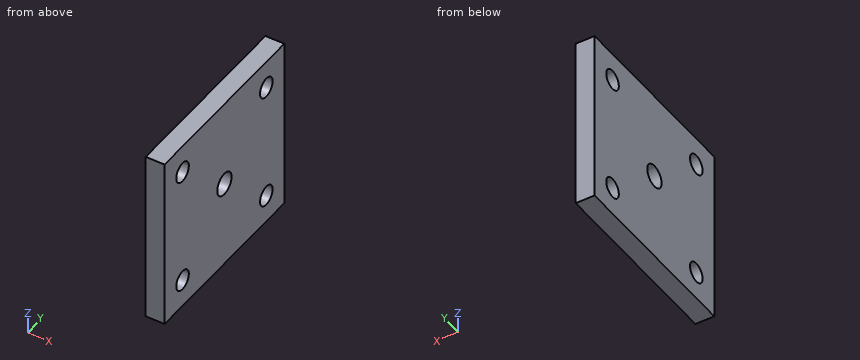
from build123d import *

# Parameters (mm, degrees)
F0_W     = 100
F0_H     = 93
F1_DEPTH = 10
F3_D     = 10.5
F4_D     = 12


with BuildPart() as f1:
    # F0 (on Right) → F1 (new body)
    with BuildSketch(Plane.YZ):
        with Locations((8.67743, 4.971333)):
            Rectangle(F0_W, F0_H)
    extrude(amount=F1_DEPTH)

    # F3 (through all)
    with Locations(Plane.YZ.offset(10)):
        with Locations((-26.32257, 36.471333), (43.67743, 36.471333), (-26.32257, -26.528667), (43.67743, -26.528667)):
            Hole(F3_D / 2)

    # F4 (through all)
    with Locations(Plane.YZ.offset(10)):
        with Locations((8.67743, 4.971333)):
            Hole(F4_D / 2)


solid = f1.part
Read the model definition and answer for the solid it produces. Units are mm, in the model's axes. Coordinates: 2 decimals unless noted, no trailing zeros. Order: outer loops, then holes, each group sorted by start corner. A loop starts at its lowest first (then second) coordinate and runs counter-clockwise, first axis right, second up. Notation, with made-up numbers: M -12,9 L 31,9 A13 cw 31,28 Z; hole C 87.25,70.5 d4. An arc over 180 degrees is marked long. Put each result on its own line as item: value. Start each with the question number.
Item 1: Section C-C, the plane x = 5.5 is taken. Determine the outline of the cut face in (y, z).
Item 2: Consider probe 1 along Y at (x, z) = (6, 37); probe 2 along Z at (x, y) = (7.25, 42); probe 3 along Y at (x, z) = (2.25, -28). Determine where each line is inside the solid, lowest interval first. Write a range as [from, to].
Item 3: Section A-A, the plane y = 40 is taken. Determine the outline of the cut face in (x, z).
Item 4: Section D-D, the plane y = 7.5 is taken. Determine the outline of the cut face in (x, z), plus the area to 3 significant figures.
Item 5: Section B-B, the plane z = 39.5 is taken. Determine the outline of the cut face in (x, y).
Computed:
1. outline: M -41.32,-41.53 L 58.68,-41.53 L 58.68,51.47 L -41.32,51.47 Z; hole C -26.32,-26.53 d10.5; hole C -26.32,36.47 d10.5; hole C 8.68,4.97 d12; hole C 43.68,-26.53 d10.5; hole C 43.68,36.47 d10.5
2. probe 1: y = [-41.32, -31.55], [-21.1, 38.45], [48.9, 58.68]
2. probe 2: z = [-41.53, -31.5], [-21.55, 31.5], [41.45, 51.47]
2. probe 3: y = [-41.32, -31.36], [-21.28, 38.64], [48.72, 58.68]
3. outline: M 0,-41.53 L 10,-41.53 L 10,-30.28 L 0,-30.28 Z; M 0,-22.78 L 10,-22.78 L 10,32.72 L 0,32.72 Z; M 0,40.22 L 10,40.22 L 10,51.47 L 0,51.47 Z
4. outline: M 0,-41.53 L 10,-41.53 L 10,-0.91 L 0,-0.91 Z; M 0,10.85 L 10,10.85 L 10,51.47 L 0,51.47 Z
4. area: 812 mm2
5. outline: M 0,-41.32 L 10,-41.32 L 10,-30.61 L 0,-30.61 Z; M 0,-22.03 L 10,-22.03 L 10,39.39 L 0,39.39 Z; M 0,47.97 L 10,47.97 L 10,58.68 L 0,58.68 Z
